Geometry check sheet. Reference: the model listing, model coordinates, mm. A direction names the side the tool comes from. Round coordinates to 2 decimals unless told otherwise and drop trailing zeros. Loops run counter-clockwise (first coordinate to the right, second up) from the corner with the lowest first, then second, coordinate; pieces in that order, holes last. Notation, with made-up numbers: M 69,86.5 L 116,86.5 A11 cw 116,95.5 Z; hole C 35,-28 d11. An arc over 180 degrees is marked long. Use one line per item in the form item = value. Start each with the question number.
1. Go/stop test with flat-tipped pins: pin 1 (2 mm diameter, centred on x = -30.5, z = 0.5, fed in from -Y); pin 2 (3.5 mm diameter, centred on y = -4, z = -1.5, fed in from -X); pin 3 (1.5 mm diameter, centred on x = -36, y = 9.5, fed in from -Z). Record where each tip stops, or that it passes through.
2. Material ranges on line 1 (Y direction, x = 40, z = -0.75); line 2 (X direction, y = -0.75, z = -0.5); line 3 (X direction, y = -1.25, z = -1.75), recorded low to high.
3. Draft check along X on faces 1 (the cylindrical face through (27, 0, 1)), 2 (the flat face through (45, 0, 1)), 3 (the flat face through (28, 0, -3)). Enter one of: pulls with the +X half, pulls with the -X half, needs draft (parallel to the pull), parting line crosses it, or undercut.
4. Set-up check for faces 4 (the flat face through (11.377, 0, -1)), 5 (the cylindrical face through (42, 0, 1)): record each of +Z, -Z, +X, -X, +Y, -Y from which the full face is reachable in a straight line by a thin tool's end or side.
5. Cross-section at D-D (x = -2). Record the boundary of the cut face in (y, z).
6. Cross-section at C-C (x = 25). Record the boundary of the cut face in (y, z).
7. Cross-section at B-B (z = 2). Record the boundary of the cut face in (x, y).
8. Cross-section at A-A (y = 0). Record the boundary of the cut face in (x, z).
```python
from build123d import *

# Parameters (mm, degrees)
BOSS_EXTRUDE2_DEPTH = 5
SKETCH3_R           = 2
CUT_EXTRUDE1_DEPTH  = 48.696960071
SKETCH5_W           = 33.623135457
SKETCH5_H           = 30
BOSS_EXTRUDE3_DEPTH = 3
SKETCH6_R           = 2
CUT_EXTRUDE2_DEPTH  = 3
SKETCH7_R           = 2
CUT_EXTRUDE3_DEPTH  = 49.104053883


with BuildPart() as part:
    # Sketch1 → Boss-Extrude2 (new body)
    with BuildSketch(Plane.XY):
        with BuildLine():
            Line((-30, 15), (45, 15))
            Line((45, 15), (45, -15))
            Line((45, -15), (-30, -15))
            ThreePointArc((-30, -15), (-45, 0), (-30, 15))
        make_face()
    extrude(amount=BOSS_EXTRUDE2_DEPTH)

    # Sketch3 → Cut-Extrude1 (cut, through all)
    with BuildSketch(Plane(origin=(0, 0, 0), x_dir=(-1, 0, 0), z_dir=(0, 0, -1))):
        with Locations((-40, 0)):
            Circle(SKETCH3_R)
        with Locations((-25, 0)):
            Circle(SKETCH3_R)
    extrude(amount=-CUT_EXTRUDE1_DEPTH, mode=Mode.SUBTRACT)

    # Sketch5 → Boss-Extrude3 (add)
    with BuildSketch(Plane(origin=(0, 0, 0), x_dir=(-1, 0, 0), z_dir=(0, 0, -1))):
        with Locations((-28.188432271, 0)):
            Rectangle(SKETCH5_W, SKETCH5_H)
    extrude(amount=BOSS_EXTRUDE3_DEPTH)

    # Sketch6 → Cut-Extrude2 (cut)
    with BuildSketch(Plane(origin=(0, 0, -3), x_dir=(-1, 0, 0), z_dir=(0, 0, -1))):
        with Locations((-40, 0)):
            Circle(SKETCH6_R)
        with Locations((-25, 0)):
            Circle(SKETCH6_R)
    extrude(amount=-CUT_EXTRUDE2_DEPTH, mode=Mode.SUBTRACT)

    # Sketch7 → Cut-Extrude3 (cut, through all)
    with BuildSketch(Plane.XY.offset(5)):
        with Locations((-30, 0)):
            Circle(SKETCH7_R)
    extrude(amount=-CUT_EXTRUDE3_DEPTH, mode=Mode.SUBTRACT)


solid = part.part
```
Reported:
q1.pin_1 = -15
q1.pin_2 = -44.68
q1.pin_3 = 0
q2.line_1 = -15 to -2, 2 to 15
q2.line_2 = 11.38 to 23.15, 26.85 to 38.15, 41.85 to 45
q2.line_3 = 11.38 to 23.44, 26.56 to 38.44, 41.56 to 45
q3.face_1 = undercut
q3.face_2 = pulls with the +X half
q3.face_3 = needs draft
q4.face_4 = -Z, -X, +Y, -Y
q4.face_5 = +Z, -Z
q5.outline = M -15,0 L 15,0 L 15,5 L -15,5 Z
q6.outline = M -15,-3 L -2,-3 L -2,5 L -15,5 Z; M 2,-3 L 15,-3 L 15,5 L 2,5 Z
q7.outline = M -30,-15 L 45,-15 L 45,15 L -30,15 A15 ccw Z; hole C -30,0 d4; hole C 25,0 d4; hole C 40,0 d4
q8.outline = M -45,0 L -32,0 L -32,5 L -45,5 Z; M -28,0 L 11.38,0 L 11.38,-3 L 23,-3 L 23,5 L -28,5 Z; M 27,-3 L 38,-3 L 38,5 L 27,5 Z; M 42,-3 L 45,-3 L 45,5 L 42,5 Z
